Autodesk Inventor part; units mm, degrees
ref_plane "YZ Plane" through (0, 0, 0) normal (1, 0, 0) x (0, 1, 0)
ref_plane "XZ Plane" through (0, 0, 0) normal (0, 1, 0) x (-1, 0, 0)
ref_plane "XY Plane" through (0, 0, 0) normal (0, 0, 1) x (1, 0, 0)
sketch "Sketch1" plane through (0, 0, 0) normal (0, 1, 0) x (-1, 0, 0)
  line L0 (0, 0) -> (50, 0)
  line L1 (50, 0) -> (50, -40)
  line L2 (50, -40) -> (0, -40)
  line L3 (0, -40) -> (0, 0)
  line L4 (0, -5) -> (-41, -5)
  line L5 (-41, -5) -> (-41, -10)
  line L6 (-41, -10) -> (0, -10)
  line L7 (0, -10) -> (0, -5)
  line L8 (0, -30) -> (-41, -30)
  line L9 (-41, -30) -> (-41, -35)
  line L10 (-41, -35) -> (0, -35)
  line L11 (0, -35) -> (0, -30)
  line L12 (0, 0) -> (-3, 0)
  line L13 (-3, 0) -> (-3, -5)
  line L14 (-3, -5) -> (0, -5)
  line L15 (0, -5) -> (0, 0)
  line L16 (0, -40) -> (-3, -40)
  line L17 (-3, -40) -> (-3, -35)
  line L18 (-3, -35) -> (0, -35)
  line L19 (0, -35) -> (0, -40)
  line L20 (0, -10) -> (-21, -10)
  line L21 (-21, -10) -> (-21, -30)
  line L22 (-21, -30) -> (0, -30)
  line L23 (0, -30) -> (0, -10)
  point P0 (0, -10)
  point P1 (-21, -10)
  dimension "d0" = 50
  dimension "d1" = 40
  dimension "d2" = 41
  dimension "d3" = 41
  dimension "d4" = 5
  dimension "d5" = 5
  dimension "d6" = 5
  dimension "d7" = 5
  dimension "d8" = 3
  dimension "d9" = 5
  dimension "d39" = 21
extrude "Extrusion1" add sketch "Sketch1" along normal blind 20
sketch "Sketch2" plane through (0, 20, 0) normal (0, 1, 0) x (1, 0, 0)
  line L0 (-50, 40) -> (-50, 0)
  line L1 (-50, 5) -> (0, 5)
  line L2 (0, 5) -> (0, 35)
  line L3 (0, 35) -> (-50, 35)
  line L4 (-50, 35) -> (-50, 5)
  line L5 (3, 40) -> (-50, 40)
  point P0 (0, 0)
  point P1 (-50, 35)
  dimension "d12" = 50
  dimension "d13" = 30
  dimension "d26" = 5
extrude "Extrusion2" cut sketch "Sketch2" against normal blind 15
sketch "Sketch3" plane through (3, 0, -5) normal (0, 0, 1) x (1, 0, 0)
  circle A0 centre (28, 10) radius 3.5
  line L0 (38, 0) -> (38, 20)
  line L1 (0, 20) -> (38, 20)
  point P0 (-3, 0)
  point P1 (19, 20)
  dimension "d16" = 10
  dimension "d17" = 10
  dimension "d20" = 7
extrude "Extrusion3" cut sketch "Sketch3" against normal blind 4
sketch "Sketch4" plane through (41, 0, -35) normal (0, 0, -1) x (-1, 0, 0)
  circle A0 centre (10, 10) radius 3.5
  circle A1 centre (10, 10) radius 3.5
  point P0 (41, 0)
extrude "Extrusion4" cut sketch "Sketch4" against normal blind 4
sketch "Sketch5" plane through (31, 10, -31) normal (0, 0, -1) x (-1, 0, 0)
  circle A0 centre (0, 0) radius 2
  point P0 (31, -10)
  dimension "d23" = 4
extrude "Extrusion5" cut sketch "Sketch5" against normal through all
sketch "Sketch6" plane through (0, 0, 0) normal (0, -1, 0) x (1, 0, 0)
  circle A0 centre (-25, -17.5) radius 3.5
  line L0 (0, -5) -> (-50, -5)
  point P0 (0, 0)
  point P1 (-50, -35)
  point P2 (0, -35)
  dimension "d27" = 7
  dimension "d29" = 25
  dimension "d44" = 12.5
extrude "Extrusion6" cut sketch "Sketch6" against normal blind 4
sketch "Sketch7" plane through (-25, 4, -17.5) normal (0, -1, 0) x (1, 0, 0)
  circle A0 centre (0, 0) radius 2
  point P0 (25, 17.5)
  dimension "d32" = 4
extrude "Extrusion7" cut sketch "Sketch7" against normal blind 4
sketch "Sketch9" plane through (0, 20, 0) normal (0, 1, 0) x (1, 0, 0)
  line L0 (3, 35) -> (3, 40)
  line L1 (-50, 35) -> (0, 35)
  line L2 (3, 40) -> (-17, 40)
  line L3 (-17, 40) -> (-17, 35)
  line L4 (-17, 35) -> (3, 35)
  line L5 (3, 35) -> (3, 40)
  line L6 (0, 35) -> (0, 5)
  line L7 (3, 35) -> (0, 35)
  line L8 (0, 35) -> (0, 25)
  line L9 (0, 25) -> (3, 25)
  line L10 (3, 25) -> (3, 35)
  point P0 (0, 0)
  point P1 (0, 15)
  dimension "d40" = 20
  dimension "d41" = 10
extrude "Extrusion9" add sketch "Sketch9" along normal blind 75
properties part number "PowerSupplyAttachTop"
Model file for the job. Use its own axes, mm. A direction names the side the tool comes from. Coordinates: 2 decimals unless noted, no trailing zeros. Order: outer loops, then holes, each group sorted by start corner. A loop starts at its lowest first (then second) coordinate and runs counter-clockwise, first axis right, second up. Notation, with made-up numbers: (-15.75, 88) - (25.25, 88) arc R28 ccw to (25.25, 107) - close; hole circle Ø3 at (36.5, -0.75). An arc over 180 degrees is marked (long way). Return JSON: item names as keys, results as strings. Group by question number.
1) Mould opens along Y. For faces 1 (the flat face through (3, 57, -33)), 2 (the flat face through (-33, 20, -37)), 3 (the cylindrical face through (29.092, 10.601, -30.507)), 4 (the flat face through (-23, 4, -19)) say: released by +Y, released by -Y, zero draft, split by the parting line, or undercut.
2) Saw through at D-D, the plane x = -9.5. Write the cut outline in (y, z).
3) Saw through at C-C, the plane z = -17.5. Write the cut outline in (x, y).
4) Probe line 1 (Z direction, x = -38, y = 15.5); line 2 (Z direction, x = -25, y = 4.3); line 3 (Y direction, x = 31, z = -6.6). List the from-to ranges inside material, lowest first. Write a range as from..to.
5) Tool access for faces 5 (the cylindrical face through (29.385, 6.895, -33.028)), 6 (the flat face through (33, 8, -9)), 7 (the flat face through (33.4, 9.9, -10)), 8 (the flat face through (-14, 41, -35)): list every direction of +Z, -Z, +X, -X, +Y, -Y with a clear straight run to the whole face (end or side of a thin tool).
6) Saw through at A-A, the plane x = 24. Write the cut outline in (y, z), plus the area to 3 significant figures.
7) Flat gauge pins, fed straight in: P1, Ø6.5, axis at x = 31, y = 10, coming from the +Z side; P2, Ø8, axis at x = 31, y = 10, coming from the -Z side; P3, Ø2, axis at y = 47.5, z = -30, coming from the +X side. Where does each tip first touch, or does it go through?
8) Saw through at B-B, the plane y = 10. Count the separate pieces of the cut face and the enclosed holes in it, plus the area to 3 significant figures.
Values found:
{
 "1": {"face 1": "zero draft", "face 2": "released by +Y", "face 3": "undercut", "face 4": "released by -Y"},
 "2": {"outline": "(0, -40) - (95, -40) - (95, -35) - (5, -35) - (5, -5) - (20, -5) - (20, 0) - (0, 0) - close"},
 "3": {"outline": "(-50, 0) - (-28.5, 0) - (-28.5, 4) - (-27, 4) - (-27, 5) - (-50, 5) - close; (-23, 4) - (-21.5, 4) - (-21.5, 0) - (21, 0) - (21, 20) - (0, 20) - (0, 5) - (-23, 5) - close"},
 "4": {"line 1": "z = -40..-35, -5..0", "line 2": "z = -40..-19.5, -15.5..0", "line 3": "y = 0..6.5, 13.5..20"},
 "5": {"face 5": "-Z", "face 6": "+Z", "face 7": "+X, +Y, -Y", "face 8": "-X, +Y"},
 "6": {"outline": "(0, -35) - (20, -35) - (20, -30) - (0, -30) - close; (0, -10) - (20, -10) - (20, -5) - (0, -5) - close", "area": "200 mm²"},
 "7": {"P1": "stops at z = -9", "P2": "stops at z = -35", "P3": "stops at x = 3"},
 "8": {"separate pieces": "3", "enclosed holes": "0", "area": "1,300 mm²"}
}
